Read the model definition and answer for the solid it produces. Units are mm, in the model's axes. A direction names the side the tool comes from. Round coordinates to 2 decimals unless told otherwise and drop trailing zeros. Loops run counter-clockwise (first coordinate to the right, second up) from the corner with the lowest first, then second, coordinate; pieces in that order, holes last. Notation, with made-up numbers: (56, 21) -> (89, 21) arc R31 ccw to (89, 60) -> close; hole circle Ø2 at (-21.5, -23). An arc over 180 degrees is marked (long way). Put each result on its own line as item: value.
from build123d import *

# Parameters (mm, degrees)
EXTRUDE_1_DEPTH     = 20
SKETCH_2_R          = 2.65
CUT_EXTRUDE_1_DEPTH = 20
CUT_EXTRUDE_2_DEPTH = 4
SKETCH_5_R          = 3.2
CUT_EXTRUDE_3_DEPTH = 56


with BuildPart() as part:
    # 草图1 → 凸台-拉伸1 (new body)
    with BuildSketch(Plane.XY):
        with BuildLine():
            Line((17, -0.197530864), (1.5, -0.197530864))
            Line((1.5, -0.197530864), (1.5, -12.098431802))
            ThreePointArc((1.5, -12.098431802), (0, -34.397530864), (-1.5, -12.098431802))
            Line((-1.5, -12.098431802), (-1.5, -0.197530864))
            Line((-1.5, -0.197530864), (-17, -0.197530864))
            Line((-17, -0.197530864), (-17, -45.197530864))
            Line((-17, -45.197530864), (-32, -45.197530864))
            Line((-32, -45.197530864), (-32, -55.197530864))
            Line((-32, -55.197530864), (32, -55.197530864))
            Line((32, -55.197530864), (32, -45.197530864))
            Line((32, -45.197530864), (17, -45.197530864))
            Line((17, -45.197530864), (17, -0.197530864))
        make_face()
    extrude(amount=EXTRUDE_1_DEPTH)

    # 草图2 → 切除-拉伸1 (cut, symmetric)
    with BuildSketch(Plane(origin=(0, 0, 0), x_dir=(0, 0, -1), z_dir=(1, 0, 0))):
        with Locations((-10, -6.697530864)):
            Circle(SKETCH_2_R)
    extrude(amount=CUT_EXTRUDE_1_DEPTH, both=True, mode=Mode.SUBTRACT)

    # 草图3 → 切除-拉伸2 (cut)
    with BuildSketch(Plane(origin=(17, 0, 0), x_dir=(0, 0, -1), z_dir=(1, 0, 0))):
        Polygon((-5.150756421, -6.697530864), (-7.575378211, -2.497962736), (-12.424621789, -2.497962736), (-14.849243579, -6.697530864), (-12.424621789, -10.897098992), (-7.575378211, -10.897098992), align=None)
    extrude(amount=-CUT_EXTRUDE_2_DEPTH, mode=Mode.SUBTRACT)

    # 草图5 → 切除-拉伸3 (cut, through all)
    with BuildSketch(Plane.XZ.offset(55.197530864)):
        with Locations((-24.5, 10)):
            Circle(SKETCH_5_R)
        with Locations((24.5, 10)):
            Circle(SKETCH_5_R)
    extrude(amount=-CUT_EXTRUDE_3_DEPTH, mode=Mode.SUBTRACT)


solid = part.part
Item 1: The part is cut by section B-B (z = 10). State how many separate pieces and enclosed holes the cut face has, then the cut area to 3 significant figures.
Derived:
separate pieces: 5
enclosed holes: 0
area: 1,440 mm^2
Item 2: The part is cut by section A-A (x = 24.5). Determine the outline of the cut face in (y, z), then the cut area to 3 significant figures.
Derived:
outline: (-55.2, 0) -> (-45.2, 0) -> (-45.2, 6.8) -> (-55.2, 6.8) -> close; (-55.2, 13.2) -> (-45.2, 13.2) -> (-45.2, 20) -> (-55.2, 20) -> close
area: 136 mm^2
Item 3: The part is cut by section C-C (y = -22). Determine the outline of the cut face in (x, z), then the cut area to 3 significant figures.
Derived:
outline: (-17, 0) -> (-11.14, 0) -> (-11.14, 20) -> (-17, 20) -> close; (11.14, 0) -> (17, 0) -> (17, 20) -> (11.14, 20) -> close
area: 235 mm^2
Item 4: The part is cut by section D-D (z = 16). Determine the outline of the cut face in (x, y), then the cut area to 3 significant figures.
Derived:
outline: (-32, -55.2) -> (32, -55.2) -> (32, -45.2) -> (17, -45.2) -> (17, -0.2) -> (1.5, -0.2) -> (1.5, -12.1) arc R11.2 cw (long way) to (-1.5, -12.1) -> (-1.5, -0.2) -> (-17, -0.2) -> (-17, -45.2) -> (-32, -45.2) -> close
area: 1,740 mm^2
Item 5: Flat-ended cylindrical pins translate along their axes: pin 1 Ø10 at (y, z) = (-22.5, 8.5) entering from +X; pin 2 Ø12 at (x, z) = (-28, 7) entering from +Y; pin 3 Ø4 at (x, z) = (24.5, 10) entering from +Y; pin 4 Ø3 at (y, z) = (-28, 10.5) entering from -X. Find the tip coordinate at first contact, or state that the pin passes through.
Derived:
pin 1: stops at x = 17
pin 2: stops at y = -45.2
pin 3: passes through
pin 4: stops at x = -17
Item 6: Find the intervals of material crossed by line 1 along X through (y, z) = (-6, 5.5); line 2 along Z through (x, y) = (-24.5, -51); line 3 along Y through (x, z) = (14, 11.5), in increasing order.
Derived:
line 1: x = -17 to -1.5, 1.5 to 17
line 2: z = 0 to 6.8, 13.2 to 20
line 3: y = -55.2 to -10.9, -2.5 to -0.2
Item 7: Which of the six approach directions +Z, -Z, +X, -X, +Y, -Y give full straight-line access (tool end or side, diameter ignored) to faces 4 (the flat face through (1.5, -4.7, 7.6)), 5 (the flat face through (28, -45.198, 10)), 6 (the flat face through (-21, -45.198, 10)), 7 (the cylindrical face through (0.471, -34.388, 9.86)), 8 (the flat face through (15.03, -8.83, 6.38))?
Derived:
face 4: +Z, -Z, +Y
face 5: +Z, -Z, +X, +Y
face 6: +Z, -Z, -X, +Y
face 7: +Z, -Z
face 8: +X
Item 8: For a pull along X with two mould halves and no side action, classify faces 1 (the flat face through (-9, -0.198, 10)), 2 (the flat face through (-1.5, -4.9, 7.6)), 3 (the flat face through (13, -4.8, 7.9)) as pulls with the +X half, pulls with the -X half, needs draft (parallel to the pull), parting line crosses it, or undercut.
Derived:
face 1: needs draft
face 2: undercut
face 3: pulls with the +X half
